```python
from build123d import *

# Parameters (mm, degrees)
SKETCH1_W           = 60
SKETCH1_H           = 160
BOSS_EXTRUDE1_DEPTH = 5
SKETCH2_R           = 1.78
CUT_EXTRUDE1_DEPTH  = 100.9750816
SKETCH3_R           = 1.35
CUT_EXTRUDE2_DEPTH  = 100.9750816
SKETCH4_W           = 5
SKETCH4_H           = 8
CUT_EXTRUDE3_DEPTH  = 100.9750816


with BuildPart() as part:
    # Sketch1 → Boss-Extrude1 (new body)
    with BuildSketch(Plane(origin=(0, 0, 0), x_dir=(1, 0, 0), z_dir=(0, 1, 0))):
        with Locations((7.29281768, -12.624309392)):
            Rectangle(SKETCH1_W, SKETCH1_H)
    extrude(amount=BOSS_EXTRUDE1_DEPTH)

    # Sketch2 → Cut-Extrude1 (cut, through all)
    with BuildSketch(Plane(origin=(0, 5, 0), x_dir=(1, 0, 0), z_dir=(0, 1, 0))):
        with Locations(Location((-17.70718232, 62.375690608, 0), (0, 0, 270))):
            Circle(SKETCH2_R)
        with Locations(Location((32.29281768, 62.375690608, 0), (0, 0, 270))):
            Circle(SKETCH2_R)
        with Locations(Location((32.29281768, -87.624309392, 0), (0, 0, 270))):
            Circle(SKETCH2_R)
        with Locations(Location((-17.70718232, -87.624309392, 0), (0, 0, 270))):
            Circle(SKETCH2_R)
    extrude(amount=-CUT_EXTRUDE1_DEPTH, mode=Mode.SUBTRACT)

    # Sketch3 → Cut-Extrude2 (cut, through all)
    with BuildSketch(Plane(origin=(0, 5, 0), x_dir=(1, 0, 0), z_dir=(0, 1, 0))):
        with Locations(Location((25.29281768, -12.624309392, 0), (0, 0, 270))):
            Circle(SKETCH3_R)
        with Locations(Location((-10.70718232, -12.624309392, 0), (0, 0, 270))):
            Circle(SKETCH3_R)
        with Locations(Location((7.29281768, 5.375690608, 0), (0, 0, 270))):
            Circle(SKETCH3_R)
        with Locations(Location((7.29281768, -30.624309392, 0), (0, 0, 270))):
            Circle(SKETCH3_R)
    extrude(amount=-CUT_EXTRUDE2_DEPTH, mode=Mode.SUBTRACT)

    # Sketch4 → Cut-Extrude3 (cut, through all)
    with BuildSketch(Plane(origin=(0, 5, 0), x_dir=(1, 0, 0), z_dir=(0, 1, 0))):
        with Locations((-5.20718232, 33.375690608)):
            Rectangle(SKETCH4_W, SKETCH4_H)
        with Locations((19.79281768, 33.375690608)):
            Rectangle(SKETCH4_W, SKETCH4_H)
        with Locations((19.79281768, -58.624309392)):
            Rectangle(SKETCH4_W, SKETCH4_H)
        with Locations((-5.20718232, -58.624309392)):
            Rectangle(SKETCH4_W, SKETCH4_H)
    extrude(amount=-CUT_EXTRUDE3_DEPTH, mode=Mode.SUBTRACT)


solid = part.part
```
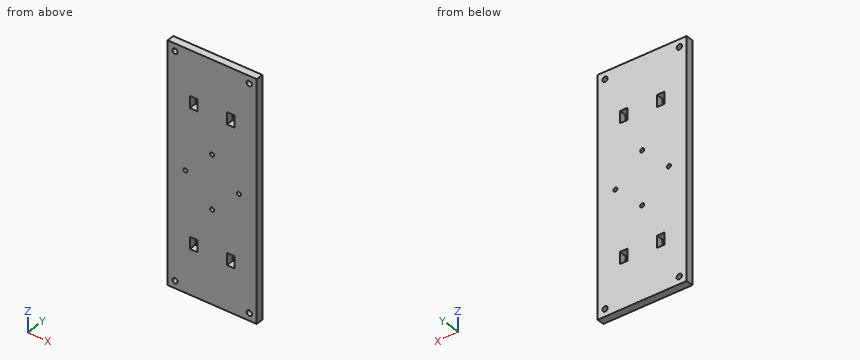
Verification items for the finished model (mm, model axes). Give positions to 0.01 mm unless a question says otherwise; leave off trailing zeros. Loops run counter-clockwise (first coordinate to the right, second up) from the corner with the lowest first, then second, coordinate; pieces in that order, holes last. Notation, with made-up numbers: M 21,22.5 L 33,22.5 A22 ccw 33,55.5 Z; hole C 46,83 d1. An arc over 180 degrees is marked long. Return JSON: item names as keys, results as strings.
1) Section check B-B, the plane y = 3.65. Count the separate pieces of the cut face and the enclosed holes in it, and give its area (3 significant figures).
Findings:
{"separate pieces": "1", "enclosed holes": "12", "area": "9,380 mm2"}
2) Material ranges on L1, parallel to Z at x = 32, y = 3; L2, parallel to Z at x = 21, y = 2.6; L3, parallel to X at y = 0.9, z = -35, recorded low to high. Write a range as [from, to].
Findings:
{"L1": "z = [-67.38, -64.13], [-60.62, 85.87], [89.38, 92.62]", "L2": "z = [-67.38, -37.38], [-29.38, 54.62], [62.62, 92.62]", "L3": "x = [-22.71, -7.71], [-2.71, 17.29], [22.29, 37.29]"}
3) Section check A-A, the plane x = -5. Enter the section's corners in (y, z), and give its area (3 significant figures).
Findings:
{"outline": "M 0,-67.38 L 5,-67.38 L 5,-37.38 L 0,-37.38 Z; M 0,-29.38 L 5,-29.38 L 5,54.62 L 0,54.62 Z; M 0,62.62 L 5,62.62 L 5,92.62 L 0,92.62 Z", "area": "720 mm2"}
